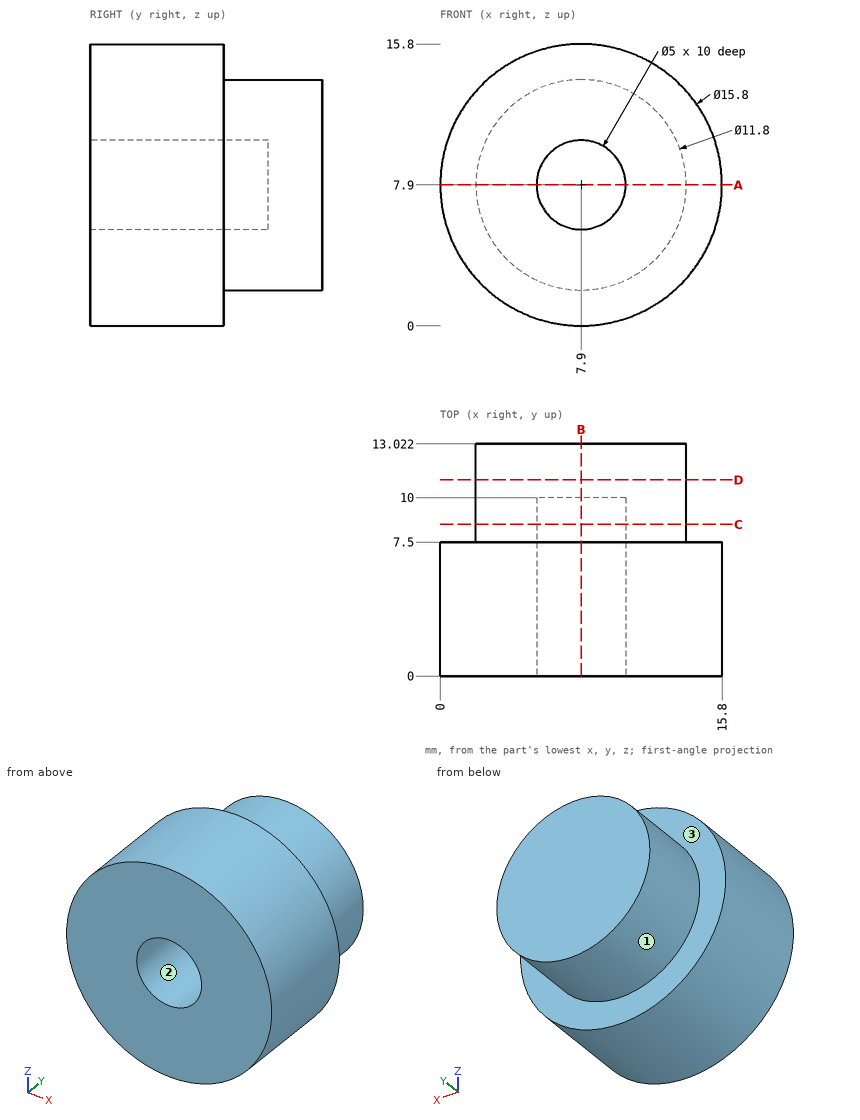
Geometry: see drawing. Coordinates: mm, zero at the bounding-box minimum. Coordinates: 2 decimals unless noted, no trailing zeros. Order: outer loops, then holes, each group sorted by start corner. A loop starts at its lowest first (then second) coordinate and runs counter-clockwise, first axis right, second up. Notation, with made-up numbers: (20, 73.25) - (64, 73.25) arc R19 cw to (64, 79.25) - close; hole circle Ø5 at (3.25, -18.75). An arc over 180 degrees is marked (long way). Write each question's results on one line, items separated by ' | '.
(1) Section query B-B, the plane x = 7.9. Return the cut outline in (y, z), plus the area to 3 significant figures.
Values found:
outline: (0, 0) - (7.5, 0) - (7.5, 2) - (13.02, 2) - (13.02, 13.8) - (7.5, 13.8) - (7.5, 15.8) - (0, 15.8) - (0, 10.4) - (10, 10.4) - (10, 5.4) - (0, 5.4) - close | area: 134 mm²
(2) Section query D-D, the plane y = 11. Return the cut outline in (x, z).
Values found:
outline: circle Ø11.8 at (7.9, 7.9)
(3) Mould query, pull axis Z, two halves, no side actions, for the marked faces 1, 2 and 3. Classes: +Z half, -Z half, draft (parallel to the pull), parting line (faces both ways), or undercut.
Values found:
face 1: parting line | face 2: undercut | face 3: draft
(4) First-contact query: pin 1 Ø5 at (x, y) = (4, 2.5) entering from -Z (1 decimal); pin 2 Ø3 at (x, y) = (12, 6) entering from +Z; pin 3 Ø5 at (y, z) = (6, 14) entering from +X. Flat tips, straight axial feed; report the tip coordinate or a pass-through.
Values found:
pin 1: stops at z = 0.1 | pin 2: stops at z = 15.36 | pin 3: stops at x = 14.93
(5) Section query A-A, the plane z = 7.9. Return the cut outline in (x, y).
Values found:
outline: (0, 0) - (5.4, 0) - (5.4, 10) - (10.4, 10) - (10.4, 0) - (15.8, 0) - (15.8, 7.5) - (13.8, 7.5) - (13.8, 13.02) - (2, 13.02) - (2, 7.5) - (0, 7.5) - close
(6) Line query: line 1 (X direction, y = 4, z = 8); line 2 (Y direction, x = 15.25, z = 6); line 3 (Y direction, x = 9.25, z = 7). Output: solid intervals per line, ascending. Write a range as [from, to].
Values found:
line 1: x = [0, 5.4], [10.4, 15.8] | line 2: y = [0, 7.5] | line 3: y = [10, 13.02]
(7) Section query C-C, the plane y = 8.5. Return the cut outline in (x, z).
Values found:
outline: circle Ø11.8 at (7.9, 7.9); hole circle Ø5 at (7.9, 7.9)
